Geometry check sheet. Reference: the model listing, model coordinates, mm. Round coordinates to 2 decimals unless told otherwise and drop trailing zeros. Order: outer loops, then holes, each group sorted by start corner. A loop starts at its lowest first (then second) coordinate and runs counter-clockwise, first axis right, second up.
(1) Cross-section at B-B on x = 10. Enter the section's corners in (y, z).
(2) Thickness scan on L1, parallel to Y at x = 70, z = -1.05; L2, parallel to X at y = 11, z = -0.2; L3, parallel to X at y = 80, z = -0.4. Record the ranges inside material, lowest first.
(3) Gauge pin test, flat end, axial feed: P1, Ø5.5, axis at x = 70, y = 80, coming from the -Z side. Record the tip position at first contact, or that the pin passes through.
(4) Cross-section at A-A on y = 20. Enter the section's corners in (x, z), and give its area (3 significant figures).
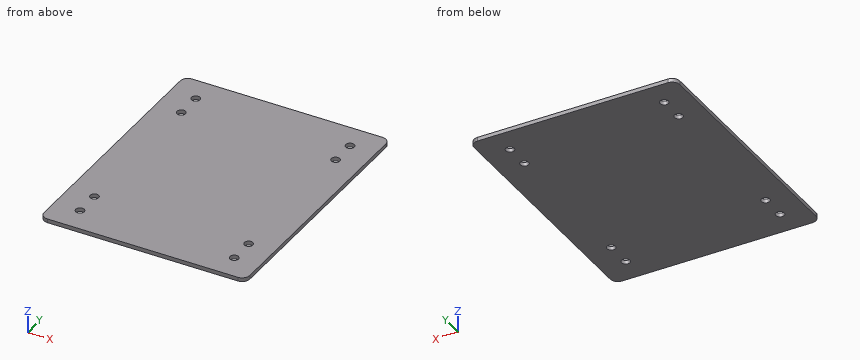
from build123d import *

# Parameters (mm, degrees)
CONVERT_SOLID1_START     = -1.5
CONVERT_SOLID1_OUTLINE_R = 1.65
CONVERT_SOLID1_DEPTH     = 1.5


# Read off the part's stored shape, not the designer's step: Convert-Solid1
with BuildPart() as part:
    # Convert-Solid1 outline → Convert-Solid1 (new body)
    with BuildSketch(Plane.XY.offset(CONVERT_SOLID1_START)):
        with BuildLine():
            Line((80, 3), (80, 97))
            ThreePointArc((80, 97), (79.121320344, 99.121320344), (77, 100))
            Line((77, 100), (3, 100))
            ThreePointArc((3, 100), (0.878679656, 99.121320344), (0, 97))
            Line((0, 97), (0, 3))
            ThreePointArc((0, 3), (0.878679656, 0.878679656), (3, 0))
            Line((3, 0), (77, 0))
            ThreePointArc((77, 0), (79.121320344, 0.878679656), (80, 3))
        make_face()
        with Locations((10, 10)):
            Circle(CONVERT_SOLID1_OUTLINE_R, mode=Mode.SUBTRACT)
        with Locations((10, 20)):
            Circle(CONVERT_SOLID1_OUTLINE_R, mode=Mode.SUBTRACT)
        with Locations((70, 10)):
            Circle(CONVERT_SOLID1_OUTLINE_R, mode=Mode.SUBTRACT)
        with Locations((70, 20)):
            Circle(CONVERT_SOLID1_OUTLINE_R, mode=Mode.SUBTRACT)
        with Locations((10, 80)):
            Circle(CONVERT_SOLID1_OUTLINE_R, mode=Mode.SUBTRACT)
        with Locations((10, 90)):
            Circle(CONVERT_SOLID1_OUTLINE_R, mode=Mode.SUBTRACT)
        with Locations((70, 80)):
            Circle(CONVERT_SOLID1_OUTLINE_R, mode=Mode.SUBTRACT)
        with Locations((70, 90)):
            Circle(CONVERT_SOLID1_OUTLINE_R, mode=Mode.SUBTRACT)
    extrude(amount=CONVERT_SOLID1_DEPTH)


solid = part.part
Found:
1. outline: (0, -1.5) - (8.35, -1.5) - (8.35, 0) - (0, 0) - close; (11.65, -1.5) - (18.35, -1.5) - (18.35, 0) - (11.65, 0) - close; (21.65, -1.5) - (78.35, -1.5) - (78.35, 0) - (21.65, 0) - close; (81.65, -1.5) - (88.35, -1.5) - (88.35, 0) - (81.65, 0) - close; (91.65, -1.5) - (100, -1.5) - (100, 0) - (91.65, 0) - close
2. L1: y = 0 to 8.35, 11.65 to 18.35, 21.65 to 78.35, 81.65 to 88.35, 91.65 to 100
2. L2: x = 0 to 8.69, 11.31 to 68.69, 71.31 to 80
2. L3: x = 0 to 8.35, 11.65 to 68.35, 71.65 to 80
3. P1: stops at z = -1.5
4. outline: (0, -1.5) - (8.35, -1.5) - (8.35, 0) - (0, 0) - close; (11.65, -1.5) - (68.35, -1.5) - (68.35, 0) - (11.65, 0) - close; (71.65, -1.5) - (80, -1.5) - (80, 0) - (71.65, 0) - close
4. area: 110 mm2
